from build123d import *

# Parameters (mm, degrees)
CROQUIS1_W                   = 5.106382979
CROQUIS1_H                   = 2
SALIENTE_EXTRUIR1_DEPTH      = 3
CROQUIS2_R                   = 0.5
SALIENTE_EXTRUIR2_DEPTH      = 2.5
SALIENTE_EXTRUIR2_DEPTH_BACK = 8.5
CROQUIS3_R                   = 0.5
SALIENTE_EXTRUIR3_DEPTH      = 2.5


with BuildPart() as part:
    # Croquis1 → Saliente-Extruir1 (new body)
    with BuildSketch(Plane.XY):
        Polygon((-2, 2), (2, 2), (2, 3), (6, 3), (6, -3), (2, -3), (2, -2), (-2, -2), (-2.5, -2), (-2.5, -0.496453901), (-2.5, 0.503546099), (-2.5, 2), align=None)
        with Locations((0.55319149, 0)):
            Rectangle(CROQUIS1_W, CROQUIS1_H, mode=Mode.SUBTRACT)
    extrude(amount=SALIENTE_EXTRUIR1_DEPTH)

    # Croquis2 → Saliente-Extruir2 (add, two sides)
    with BuildSketch(Plane(origin=(0, 3, 0), x_dir=(1, 0, 0), z_dir=(0, 1, 0))) as saliente_extruir2_sk:
        with Locations((4, -1.5)):
            Circle(CROQUIS2_R)
    extrude(amount=SALIENTE_EXTRUIR2_DEPTH)
    extrude(saliente_extruir2_sk.sketch, amount=-SALIENTE_EXTRUIR2_DEPTH_BACK)

    # Croquis3 → Saliente-Extruir3 (add)
    with BuildSketch(Plane.ZY.offset(2.5)):
        with Locations((1.5, 0)):
            Circle(CROQUIS3_R)
    extrude(amount=SALIENTE_EXTRUIR3_DEPTH)


solid = part.part
The model under review builds one solid part; all positions refer to its coordinate system, in mm. A direction names the side the tool comes from. Coordinates: 2 decimals unless noted, no trailing zeros. Write each loop counter-clockwise with the first axis right and the second up, starting at its lowest first coordinate (ties: lowest second). Pieces come first, ordered by that corner, then holes. Notation, with made-up numbers: (18, 45) - (40, 45) arc R22 cw to (40, 65) - close; hole circle Ø11 at (86.5, 42). An arc over 180 degrees is marked (long way). Answer as a JSON object with one key per item and string values. Group by question number.
1. Mouldability with a two-part tool opening along X and no side actions: class faces 1 (the face through (3.106, 0, 1)), 2 (the face through (4, 4, 2)), 3 (the face through (4, 0, 0)) as pulls with the +X half, pulls with the -X half, needs draft (parallel to the pull), parting line crosses it, or undercut.
2. Add section B-B (y = 0). Give the boundary of the cut face in (x, z).
3. Machinability: for faces 4 (the face through (4, -3, 0.8)), 5 (the face through (2, 2.5, 1.5)), 6 (the face through (0, -2, 1)), 7 (the face through (1, 1, 1)), which of the approach directions +Z, -Z, +X, -X, +Y, -Y give a long, thin tool a straight path to every point of the face, cutting with its end or side? Answer none if there is none.
4. Add section A-A (z = 1.2). Give the boundary of the cut face in (x, y), plus the area to 3 significant figures.
5. To check wall thickness, follow probe 1 along Y at (x, z) = (-0.75, 1.7); probe 2 along X at (y, z) = (0.5, 0.95); probe 3 along Y at (x, z) = (3, 0.2). State the ranges of each line that lie inside material, in increasing order.
6. Add section D-D (z = 0.5). Give the boundary of the cut face in (x, y), plus the area to 3 significant figures.
7. Add section C-C (x = 4). Give the boundary of the cut face in (y, z).
8. Clearance check with flat-ended pins moving along their axes: pin 1 Ø1.5 at (x, z) = (-0.5, 2) entering from -Y; pin 2 Ø0.5 at (y, z) = (-2.5, 1.5) entering from -X; pin 3 Ø1.1 at (y, z) = (2.5, 1) entering from -X. State where each tip first meets the part, or that it passes through.
Findings:
{
 "1": {"face 1": "undercut", "face 2": "parting line crosses it", "face 3": "needs draft"},
 "2": {"outline": "(-5, 1) - (-2.5, 1) - (-2.5, 0) - (-2, 0) - (-2, 3) - (-2.5, 3) - (-2.5, 2) - (-5, 2) - close; (3.11, 0) - (6, 0) - (6, 3) - (3.11, 3) - close"},
 "3": {"face 4": "-Y", "face 5": "+Z, -Z, -X, +Y", "face 6": "+Z, -Z, -X, -Y", "face 7": "+Z, -Z"},
 "4": {"outline": "(-5, -0.4) - (-2.5, -0.4) - (-2.5, -2) - (2, -2) - (2, -3) - (3.6, -3) - (3.6, -5.5) - (4.4, -5.5) - (4.4, -3) - (6, -3) - (6, 3) - (4.4, 3) - (4.4, 5.5) - (3.6, 5.5) - (3.6, 3) - (2, 3) - (2, 2) - (-2.5, 2) - (-2.5, 0.4) - (-5, 0.4) - close; hole (-2, -1) - (3.11, -1) - (3.11, 1) - (-2, 1) - close", "area": "37.8 mm²"},
 "5": {"probe 1": "-2 to -1, 1 to 2", "probe 2": "-2.5 to -2, 3.11 to 6", "probe 3": "-3 to -1, 1 to 3"},
 "6": {"outline": "(-2.5, -2) - (2, -2) - (2, -3) - (6, -3) - (6, 3) - (2, 3) - (2, 2) - (-2.5, 2) - close; hole (-2, -1) - (3.11, -1) - (3.11, 1) - (-2, 1) - close", "area": "31.8 mm²"},
 "7": {"outline": "(-5.5, 1) - (-3, 1) - (-3, 0) - (3, 0) - (3, 1) - (5.5, 1) - (5.5, 2) - (3, 2) - (3, 3) - (-3, 3) - (-3, 2) - (-5.5, 2) - close"},
 "8": {"pin 1": "y = -2", "pin 2": "x = 2", "pin 3": "x = -2.5"}
}
